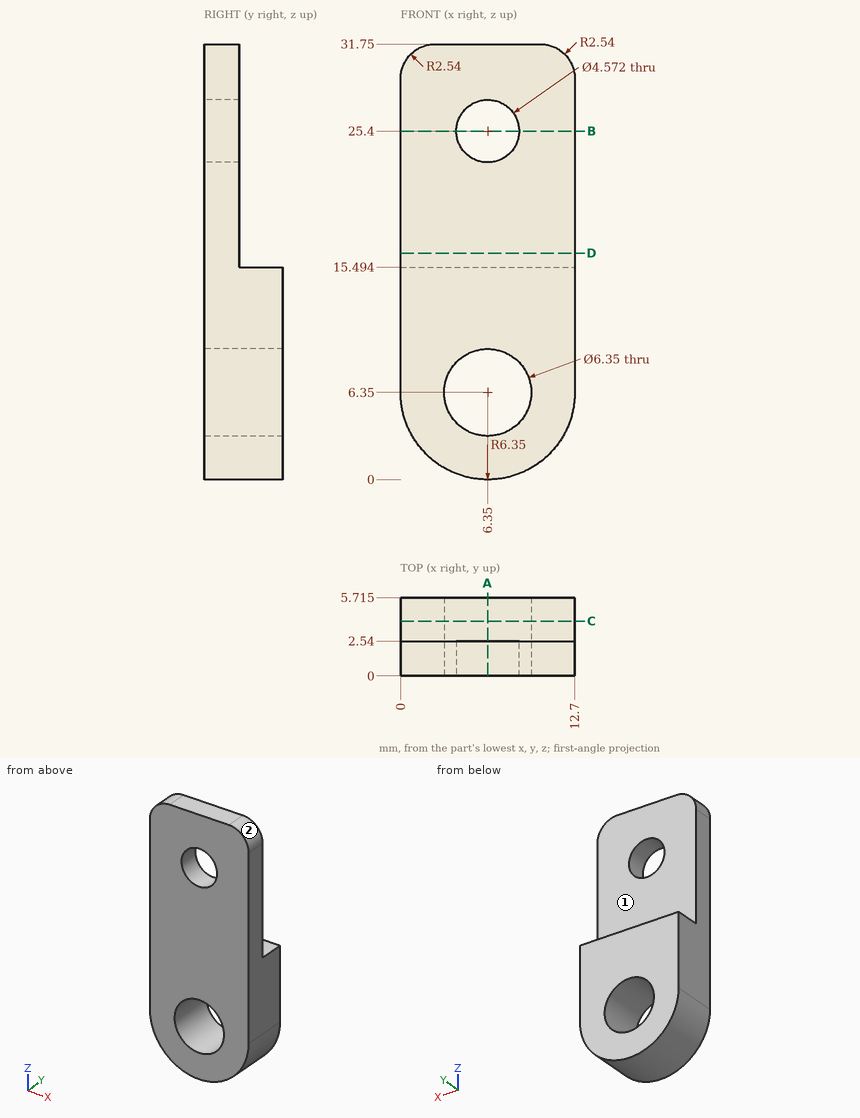
Verification items for this drawing (mm, ordinates from the low corner). A direction names the side the tool comes from. Coordinates: 2 decimals unless noted, no trailing zeros. Order: outer loops, then holes, each group sorted by start corner. A loop starts at its lowest first (then second) coordinate and runs counter-clockwise, first axis right, second up. Notation, with made-up numbers: (78.25, 45.25) - (128.25, 45.25) arc R23 cw to (128.25, 64.25) - close; hole circle Ø10 at (-32.5, 17). An arc over 180 degrees is marked (long way). Use one line per item in the form item = value.
1. Gauge pin test, flat ends, axial feed: pin 1 (3 mm diameter, centred on x = 2.5, z = 19.5, fed in from +Y); pin 2 (1.6 mm diameter, centred on x = 9.5, y = 3.5, fed in from +Z); pin 3 (6 mm diameter, centred on x = 6.35, z = 25.4, fed in from -Y). Record the tip position at first contact, or that the pin passes through.
Here are the results:
pin_1 = 2.54
pin_2 = 15.49
pin_3 = 0
2. Scan lines: line 1 (Z direction, x = 6.5, y = 0.8); line 2 (X direction, y = 1.15, z = 25.4); line 3 (Z direction, x = 6.25, y = 3.45). Record each from-to range of solid material in increasing order.
Here are the results:
line_1 = 0 to 3.18, 9.52 to 23.12, 27.68 to 31.75
line_2 = 0 to 4.06, 8.64 to 12.7
line_3 = 0 to 3.18, 9.52 to 15.49
3. Access from +Z, -Z, +X, -X, +Y, -Y to the whole of each face (thin tool, end or side, straight path). Record for the marked faces 1 and 2.
Here are the results:
face_1 = +Z, +X, -X, +Y
face_2 = +Z, +X, +Y, -Y
4. Section check C-C (y = 4). Record the boundary of the cut face in (x, z) (3 decimals).
Here are the results:
outline = (0, 6.35) arc R6.35 ccw to (12.7, 6.35) - (12.7, 15.494) - (0, 15.494) - close; hole circle Ø6.35 at (6.35, 6.35)
5. Section check D-D (z = 16.5). Record the boundary of the cut face in (x, y).
Here are the results:
outline = (0, 0) - (12.7, 0) - (12.7, 2.54) - (0, 2.54) - close
6. Section check A-A (x = 6.35). Record the boundary of the cut face in (y, z) (3 decimals).
Here are the results:
outline = (0, 0) - (5.715, 0) - (5.715, 3.175) - (0, 3.175) - close; (0, 9.525) - (5.715, 9.525) - (5.715, 15.494) - (2.54, 15.494) - (2.54, 23.114) - (0, 23.114) - close; (0, 27.686) - (2.54, 27.686) - (2.54, 31.75) - (0, 31.75) - close
7. Section check B-B (z = 25.4). Record the boundary of the cut face in (x, y).
Here are the results:
outline = (0, 0) - (4.06, 0) - (4.06, 2.54) - (0, 2.54) - close; (8.64, 0) - (12.7, 0) - (12.7, 2.54) - (8.64, 2.54) - close
